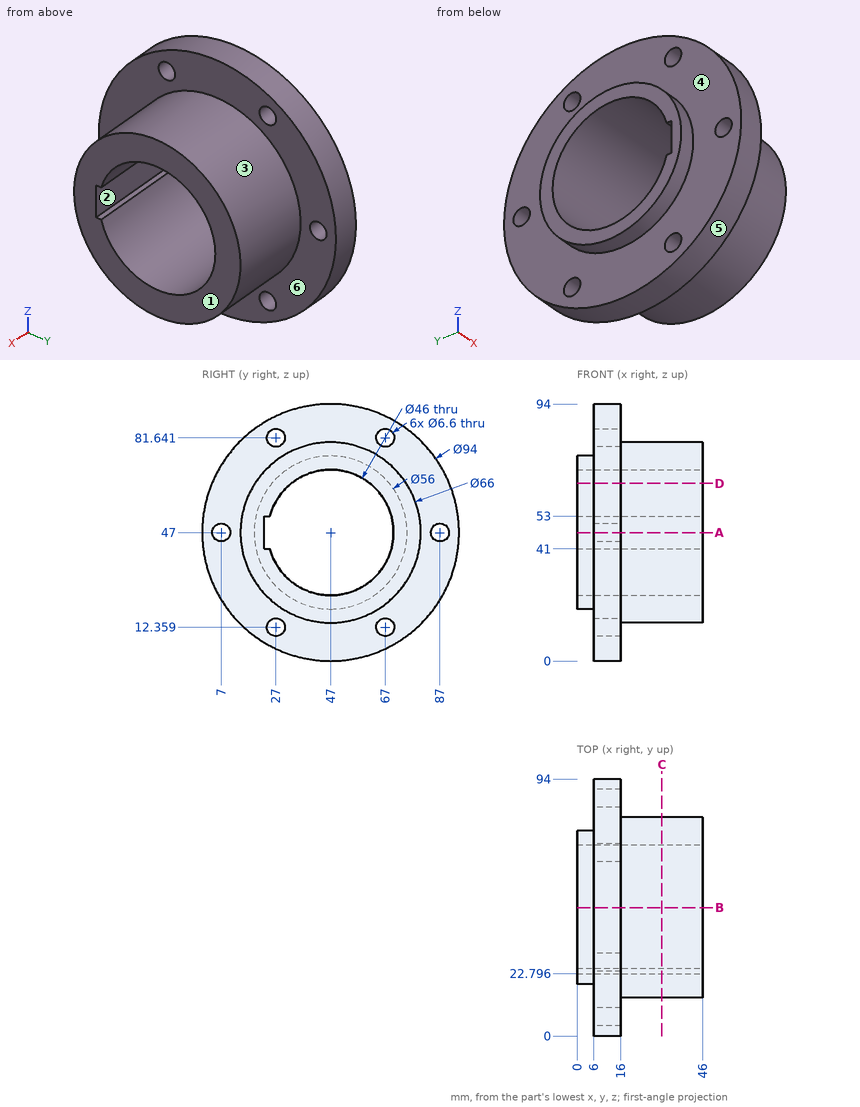
Can you work these out from the drawing? Everything is in mm from the part's minimum corner. A direction names the side the tool comes from. Round coordinates to 2 decimals unless told otherwise and drop trailing zeros. Order: outer loops, then holes, each group sorted by start corner. A loop starts at its lowest first (then second) coordinate and runs counter-clockwise, first axis right, second up. Notation, with made-up numbers: (25, -21) -> (72, -21) arc R12 cw to (72, -8) -> close; hole circle Ø6 at (14, 49). An arc over 180 degrees is marked (long way). Return JSON: item names as keys, results as strings. Group by question number.
1. I need wall thicknesses on line 1 (X direction, y = 28.5, z = 21); line 2 (X direction, y = 66, z = 86); line 3 (Z direction, x = 10, y = 31) (1 decimal). Which ranges of each line are inside material? Lowest first, please. Write a range as [from, to].
2. Will these pins go through, and if not, where does the flat tip stop? pin 1 (8.5 mm diameter, centred on y = 7, z = 47, fed in from +X); pin 2 (3 mm diameter, centred on y = 39, z = 26.5, fed in from -X); pin 3 (4 mm diameter, centred on x = 23.5, z = 38, fed in from +Y); pin 4 (0.6 mm diameter, centred on x = 24, y = 24, fed in from +Z).
3. If we section it at A-A, the plane z = 47: Write out the boundary of the cut face in (x, y).
4. If we section it at D-D, the plane z = 65: Write out the boundary of the cut face in (x, y).
5. If we section it at C-C, the plane x = 31: Write out the boundary of the cut face in (y, z), then the cut area to 3 significant figures.
6. Which directions (+Z, -Z, +X, -X, +Y, -Y) give clear straight access to the entire face, cutting with the end or side of a thin tool? Please do the marked faces 4, 5 and 6.
7. If we section it at B-B, the plane y = 47: Write out the boundary of the cut face in (x, z).
8. We'd pull the mould along Y, two halves only. Please class the marked faces 1, 2 and 3: released by +Y, released by -Y, zero draft, split by the parting line, or undercut.
Output values:
{
 "1": {"line 1": "[6, 46]", "line 2": "[6, 16]", "line 3": "[2.8, 30.5], [63.5, 91.2]"},
 "2": {"pin 1": "x = 16", "pin 2": "x = 0", "pin 3": "y = 79.25", "pin 4": "z = 70.95"},
 "3": {"outline": "(0, 19) -> (6, 19) -> (6, 10.3) -> (16, 10.3) -> (16, 14) -> (46, 14) -> (46, 22.8) -> (0, 22.8) -> close; (0, 70) -> (46, 70) -> (46, 80) -> (16, 80) -> (16, 83.7) -> (6, 83.7) -> (6, 75) -> (0, 75) -> close; (6, 0) -> (16, 0) -> (16, 3.7) -> (6, 3.7) -> close; (6, 90.3) -> (16, 90.3) -> (16, 94) -> (6, 94) -> close"},
 "4": {"outline": "(0, 25.55) -> (6, 25.55) -> (6, 3.58) -> (16, 3.58) -> (16, 19.34) -> (46, 19.34) -> (46, 32.68) -> (0, 32.68) -> close; (0, 61.32) -> (46, 61.32) -> (46, 74.66) -> (16, 74.66) -> (16, 90.42) -> (6, 90.42) -> (6, 68.45) -> (0, 68.45) -> close"},
 "5": {"outline": "circle Ø66 at (47, 47); hole (22.8, 41) -> (24.8, 41) arc R23 ccw (long way) to (24.8, 53) -> (22.8, 53) -> close", "area": "1,740 mm²"},
 "6": {"face 4": "-X", "face 5": "+X, -X", "face 6": "+X"},
 "7": {"outline": "(0, 19) -> (6, 19) -> (6, 0) -> (16, 0) -> (16, 14) -> (46, 14) -> (46, 24) -> (0, 24) -> close; (0, 70) -> (46, 70) -> (46, 80) -> (16, 80) -> (16, 94) -> (6, 94) -> (6, 75) -> (0, 75) -> close"},
 "8": {"face 1": "zero draft", "face 2": "undercut", "face 3": "split by the parting line"}
}
